CAD build for the part. Positions are in the model's coordinates, mm. Round coordinates to 2 decimals unless told otherwise and drop trailing zeros. Use one line per item in the form item = value.
from build123d import *

# Parameters (mm, degrees)
BOSS_EXTRUDE1_DEPTH = 410
SKETCH2_W           = 1200
SKETCH2_H           = 2.1
SKETCH3_W           = 1200
SKETCH3_H           = 2.1


with BuildPart() as part:
    # Sketch1 → Boss-Extrude1 (new body)
    with BuildSketch(Plane.XY):
        with BuildLine():
            Line((-9, -20), (-3, -20))
            Line((-3, -20), (-3, -18))
            Line((-3, -18), (-6, -18))
            Line((-6, -18), (-6, -17.060660172))
            Line((-6, -17.060660172), (-2.939339828, -14))
            Line((-2.939339828, -14), (-2.5, -14))
            Line((-2.5, -14), (-0.653589838, -14))
            ThreePointArc((-0.653589838, -14), (-0.524180316, -13.982962913), (-0.403589838, -13.933012702))
            Line((-0.403589838, -13.933012702), (0, -13.7))
            Line((0, -13.7), (0.403589838, -13.933012702))
            ThreePointArc((0.403589838, -13.933012702), (0.524180316, -13.982962913), (0.653589838, -14))
            Line((0.653589838, -14), (2.939339828, -14))
            Line((2.939339828, -14), (6, -17.060660172))
            Line((6, -17.060660172), (6, -18))
            Line((6, -18), (3, -18))
            Line((3, -18), (3, -20))
            Line((3, -20), (9, -20))
            ThreePointArc((9, -20), (9.707106781, -19.707106781), (10, -19))
            Line((10, -19), (10, -13))
            Line((10, -13), (8, -13))
            Line((8, -13), (8, -16))
            Line((8, -16), (7.060660172, -16))
            Line((7.060660172, -16), (4, -12.939339828))
            Line((4, -12.939339828), (4, -12.5))
            Line((4, -12.5), (4, -10.653589838))
            ThreePointArc((4, -10.653589838), (3.982962913, -10.524180316), (3.933012702, -10.403589838))
            Line((3.933012702, -10.403589838), (3.7, -10))
            Line((3.7, -10), (3.933012702, -9.596410162))
            ThreePointArc((3.933012702, -9.596410162), (3.982962913, -9.475819684), (4, -9.346410162))
            Line((4, -9.346410162), (4, -7.060660172))
            Line((4, -7.060660172), (7.060660172, -4))
            Line((7.060660172, -4), (8, -4))
            Line((8, -4), (8, -7))
            Line((8, -7), (10, -7))
            Line((10, -7), (10, 7))
            Line((10, 7), (8, 7))
            Line((8, 7), (8, 4))
            Line((8, 4), (7.060660172, 4))
            Line((7.060660172, 4), (4, 7.060660172))
            Line((4, 7.060660172), (4, 9.346410162))
            ThreePointArc((4, 9.346410162), (3.982962913, 9.475819684), (3.933012702, 9.596410162))
            Line((3.933012702, 9.596410162), (3.7, 10))
            Line((3.7, 10), (3.933012702, 10.403589838))
            ThreePointArc((3.933012702, 10.403589838), (3.982962913, 10.524180316), (4, 10.653589838))
            Line((4, 10.653589838), (4, 12.5))
            Line((4, 12.5), (4, 12.939339828))
            Line((4, 12.939339828), (7.060660172, 16))
            Line((7.060660172, 16), (8, 16))
            Line((8, 16), (8, 13))
            Line((8, 13), (10, 13))
            Line((10, 13), (10, 19))
            ThreePointArc((10, 19), (9.707106781, 19.707106781), (9, 20))
            Line((9, 20), (3, 20))
            Line((3, 20), (3, 18))
            Line((3, 18), (6, 18))
            Line((6, 18), (6, 17.060660172))
            Line((6, 17.060660172), (2.939339828, 14))
            Line((2.939339828, 14), (0.653589838, 14))
            ThreePointArc((0.653589838, 14), (0.524180316, 13.982962913), (0.403589838, 13.933012702))
            Line((0.403589838, 13.933012702), (0, 13.7))
            Line((0, 13.7), (-0.403589838, 13.933012702))
            ThreePointArc((-0.403589838, 13.933012702), (-0.524180316, 13.982962913), (-0.653589838, 14))
            Line((-0.653589838, 14), (-2.5, 14))
            Line((-2.5, 14), (-2.939339828, 14))
            Line((-2.939339828, 14), (-6, 17.060660172))
            Line((-6, 17.060660172), (-6, 18))
            Line((-6, 18), (-3, 18))
            Line((-3, 18), (-3, 20))
            Line((-3, 20), (-9, 20))
            ThreePointArc((-9, 20), (-9.707106781, 19.707106781), (-10, 19))
            Line((-10, 19), (-10, 13))
            Line((-10, 13), (-8, 13))
            Line((-8, 13), (-8, 16))
            Line((-8, 16), (-7.060660172, 16))
            Line((-7.060660172, 16), (-4, 12.939339828))
            Line((-4, 12.939339828), (-4, 10.653589838))
            ThreePointArc((-4, 10.653589838), (-3.982962913, 10.524180316), (-3.933012702, 10.403589838))
            Line((-3.933012702, 10.403589838), (-3.7, 10))
            Line((-3.7, 10), (-3.933012702, 9.596410162))
            ThreePointArc((-3.933012702, 9.596410162), (-3.982962913, 9.475819684), (-4, 9.346410162))
            Line((-4, 9.346410162), (-4, 7.5))
            Line((-4, 7.5), (-4, 7.060660172))
            Line((-4, 7.060660172), (-7.060660172, 4))
            Line((-7.060660172, 4), (-8, 4))
            Line((-8, 4), (-8, 7))
            Line((-8, 7), (-10, 7))
            Line((-10, 7), (-10, -7))
            Line((-10, -7), (-8, -7))
            Line((-8, -7), (-8, -4))
            Line((-8, -4), (-7.060660172, -4))
            Line((-7.060660172, -4), (-4, -7.060660172))
            Line((-4, -7.060660172), (-4, -7.5))
            Line((-4, -7.5), (-4, -9.346410162))
            ThreePointArc((-4, -9.346410162), (-3.982962913, -9.475819684), (-3.933012702, -9.596410162))
            Line((-3.933012702, -9.596410162), (-3.7, -10))
            Line((-3.7, -10), (-3.933012702, -10.403589838))
            ThreePointArc((-3.933012702, -10.403589838), (-3.982962913, -10.524180316), (-4, -10.653589838))
            Line((-4, -10.653589838), (-4, -12.939339828))
            Line((-4, -12.939339828), (-7.060660172, -16))
            Line((-7.060660172, -16), (-8, -16))
            Line((-8, -16), (-8, -13))
            Line((-8, -13), (-10, -13))
            Line((-10, -13), (-10, -19))
            ThreePointArc((-10, -19), (-9.707106781, -19.707106781), (-9, -20))
        make_face()
        with BuildLine():
            Line((-7.7, -2), (-7.063603897, -2))
            ThreePointArc((-7.063603897, -2), (-6.948798867, -2.02283614), (-6.851471863, -2.087867966))
            Line((-6.851471863, -2.087867966), (-2.939339828, -6))
            Line((-2.939339828, -6), (2.939339828, -6))
            Line((2.939339828, -6), (6.851471863, -2.087867966))
            ThreePointArc((6.851471863, -2.087867966), (6.948798867, -2.02283614), (7.063603897, -2))
            Line((7.063603897, -2), (7.7, -2))
            ThreePointArc((7.7, -2), (7.912132034, -1.912132034), (8, -1.7))
            Line((8, -1.7), (8, 1.7))
            ThreePointArc((8, 1.7), (7.912132034, 1.912132034), (7.7, 2))
            Line((7.7, 2), (7.063603897, 2))
            ThreePointArc((7.063603897, 2), (6.948798867, 2.02283614), (6.851471863, 2.087867966))
            Line((6.851471863, 2.087867966), (2.939339828, 6))
            Line((2.939339828, 6), (-2.939339828, 6))
            Line((-2.939339828, 6), (-6.851471863, 2.087867966))
            ThreePointArc((-6.851471863, 2.087867966), (-6.948798867, 2.02283614), (-7.063603897, 2))
            Line((-7.063603897, 2), (-7.7, 2))
            ThreePointArc((-7.7, 2), (-7.912132034, 1.912132034), (-8, 1.7))
            Line((-8, 1.7), (-8, -1.7))
            ThreePointArc((-8, -1.7), (-7.912132034, -1.912132034), (-7.7, -2))
        make_face(mode=Mode.SUBTRACT)
    extrude(amount=-BOSS_EXTRUDE1_DEPTH)

    # Sketch2 → Cut-Revolve1 (revolve, cut)
    with BuildSketch(Plane(origin=(0, 0, 0), x_dir=(0, 0, -1), z_dir=(1, 0, 0))):
        with Locations((600, 11.05)):
            Rectangle(SKETCH2_W, SKETCH2_H)
    revolve(axis=Axis((0, 10, -1200), (0, 0, 1)), mode=Mode.SUBTRACT)

    # Sketch3 → Cut-Revolve2 (revolve, cut)
    with BuildSketch(Plane(origin=(0, 0, 0), x_dir=(0, 0, -1), z_dir=(1, 0, 0))):
        with Locations((600, -8.95)):
            Rectangle(SKETCH3_W, SKETCH3_H)
    revolve(axis=Axis((0, -10, -1200), (0, 0, 1)), mode=Mode.SUBTRACT)


solid = part.part
1. Probe line 1 along Y through (x, z) = (0, -246.5); line 2 along Y through (x, z) = (7.25, -75); line 3 along Y through (x, z) = (-8.25, -227). List the from-to ranges inside material, lowest first. Write a range as from..to.
Completed:
line_1 = -13.7..-12.1, -7.9..-6, 6..7.9, 12.1..13.7
line_2 = -20..-16, -4..-2, 2..4, 16..20
line_3 = -20..-13, -7..7, 13..20
2. Drop flat-ended pins along their axis: P1, Ø0.7, axis at y = -11.5, z = -144, coming from the -X side; P2, Ø3, axis at x = -1, z = -314, coming from the +Y side. Give the stop position or say it passes through.
Completed:
P1 = -4
P2 = 14
3. Cut at A-A on z = -113.5. State how many separate pieces and enclosed holes the cut face has, and give its area (3 significant figures).
Completed:
separate_pieces = 1
enclosed_holes = 3
area = 324 mm2
